Source: CAD feature listing. Evaluate the final solid. Frame: model axes, mm. A direction names the side the tool comes from. Give positions to 0.01 mm unless a question says otherwise; leave off trailing zeros. Write each loop counter-clockwise with the first axis right and the second up, starting at its lowest first coordinate (ties: lowest second). Pieces come first, ordered by that corner, then holes. Notation, with made-up numbers: (1.25, -28.5) -> (51.25, -28.5) arc R20 cw to (51.25, -22.5) -> close; hole circle Ø9 at (-10.5, 2). An arc over 180 degrees is marked (long way). Answer as a JSON object with one key per item and string values. Group by question number.
Item 1: Section query B-B on z = 7.5. Return the cut outline in (x, y).
Item 2: Section query A-A on x = 27. Return the cut outline in (y, z), plus the area to 3 significant figures.
Item 3: Section query C-C on y = 0. Return the cut outline in (x, z).
Item 4: Pull-direction query (X, two-part tool) for faces 1 (the face through (-2, 10, 9)), 2 (the face through (129.99, -0.9, 4.44)), 3 (the face through (-129.99, 0.9, 4.44)), 4 (the face through (13.25, -24, 6)); classes: pulls with the +X half, pulls with the -X half, needs draft (parallel to the pull), parting line crosses it, or undercut.
Item 5: Section query D-D on y = 13.5. Return the cut outline in (x, z).
Item 6: Ray query, probe 1 along Y at (x, z) = (44, 4.5); probe 2 along Y at (x, z) = (66, 5.75); probe 3 along Y at (x, z) = (-9, 4.5). Return the intervals inside material, ascending. Write a range as from..to.
Item 7: Access query for faces 5 (the face through (-13.25, -24, 6)), 6 (the face through (-2, 1, 0)), 7 (the face through (68.5, -0.1, 6)). Directions: +Z, -Z, +X, -X, +Y, -Y. A direction counts if a zero-diameter tool reaches every point of the face in a straight line with its end or side. Return the directions, or none.
Item 8: First-contact query: pin 1 Ø3 at (y, z) = (-20, 5) entering from +X; pin 2 Ø1.5 at (x, z) = (-2, 7.5) entering from -Y; pin 3 Ø4 at (y, z) = (3, 8) entering from -X. Flat tips, straight axial feed; report the tip coordinate or a pass-through.
from build123d import *

# Parameters (mm, degrees)
PAD_DEPTH       = 9
POCKET_DEPTH    = 6
SKETCH002_W     = 26.5
SKETCH002_H     = 35
POCKET001_DEPTH = 6


with BuildPart() as part:
    # Sketch → Pad (new body)
    with BuildSketch(Plane.XY):
        with BuildLine():
            ThreePointArc((-89, 41), (-130, 0), (-89, -41))
            Line((-89, -41), (89, -41))
            ThreePointArc((89, -41), (130, 0), (89, 41))
            Line((-89, 41), (89, 41))
        make_face()
    extrude(amount=PAD_DEPTH)

    # Sketch001 (on Face6 of Pad) → Pocket (cut)
    with BuildSketch(Plane.XY.offset(9)):
        with BuildLine():
            ThreePointArc((-62.5, 6), (-68.5, 0), (-62.5, -6))
            Line((-62.5, -6), (62.5, -6))
            ThreePointArc((62.5, -6), (68.5, 0), (62.5, 6))
            Line((-62.5, 6), (62.5, 6))
        make_face()
    extrude(amount=-POCKET_DEPTH, mode=Mode.SUBTRACT)

    # Sketch002 (on Face5 of Pocket) → Pocket001 (cut)
    with BuildSketch(Plane.XY.offset(9)):
        with Locations((0, -23.5)):
            Rectangle(SKETCH002_W, SKETCH002_H)
    extrude(amount=-POCKET001_DEPTH, mode=Mode.SUBTRACT)


solid = part.part
Worked answers:
{
 "1": {"outline": "(-89, -41) -> (-13.25, -41) -> (-13.25, -6) -> (-62.5, -6) arc R6 cw to (-62.5, 6) -> (62.5, 6) arc R6 cw to (62.5, -6) -> (13.25, -6) -> (13.25, -41) -> (89, -41) arc R41 ccw to (89, 41) -> (-89, 41) arc R41 ccw to start"},
 "2": {"outline": "(-41, 0) -> (41, 0) -> (41, 9) -> (6, 9) -> (6, 3) -> (-6, 3) -> (-6, 9) -> (-41, 9) -> close", "area": "666 mm^2"},
 "3": {"outline": "(-130, 0) -> (130, 0) -> (130, 9) -> (68.5, 9) -> (68.5, 3) -> (-68.5, 3) -> (-68.5, 9) -> (-130, 9) -> close"},
 "4": {"face 1": "needs draft", "face 2": "pulls with the +X half", "face 3": "pulls with the -X half", "face 4": "undercut"},
 "5": {"outline": "(-127.71, 0) -> (127.71, 0) -> (127.71, 9) -> (-127.71, 9) -> close"},
 "6": {"probe 1": "-41..-6, 6..41", "probe 2": "-41..-4.87, 4.87..41", "probe 3": "6..41"},
 "7": {"face 5": "+Z, -Y", "face 6": "-Z, +X, -X, +Y, -Y", "face 7": "+Z"},
 "8": {"pin 1": "x = 125.59", "pin 2": "y = 6", "pin 3": "x = -129.99"}
}
